from build123d import *

# Parameters (mm, degrees)
F1_DEPTH = 5
F3_DEPTH = 5
F4_R     = 1


with BuildPart() as f1:
    # F0 (on Top) → F1 (new body)
    with BuildSketch(Plane.XY):
        with BuildLine():
            Line((0, 34.5), (0, 32.5))
            ThreePointArc((0, 32.5), (32.5, 0), (0, -32.5))
            Line((0, -32.5), (0, -34.5))
            ThreePointArc((0, -34.5), (34.5, 0), (0, 34.5))
        make_face()
    extrude(amount=F1_DEPTH)

    # F2 (on Top) → F3 (join)
    with BuildSketch(Plane.XY):
        with BuildLine():
            Line((37.856134, -4.425073), (36.986309, -6.22602))
            ThreePointArc((36.986309, -6.22602), (43.716406, 5.833865), (35.63118, -5.362748))
            Line((35.63118, -5.362748), (36.70016, -3.645338))
            ThreePointArc((36.70016, -3.645338), (42.749633, 4.07639), (37.856134, -4.425073))
        make_face()
    extrude(amount=F3_DEPTH)

    # F4
    f4_edges = [f1.edges().sort_by_distance(p)[0] for p in [
        (42.749633, 4.07639, 0),
        (42.749633, 4.07639, 5),
    ]]
    fillet(f4_edges, radius=F4_R)


solid = f1.part
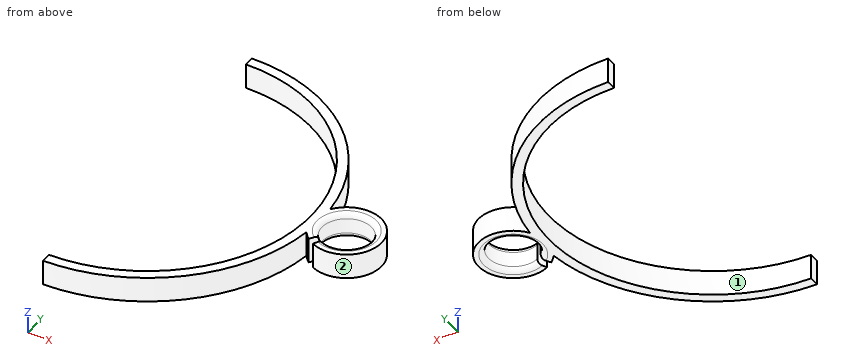
The listing builds one solid part. Answer for the finished solid, in the listing's coordinates (mm). Face numbers are marked on the shaded views. Round coordinates to 2 decimals unless told otherwise and drop trailing zeros. Write each loop counter-clockwise with the first axis right and the second up, starting at its lowest first coordinate (ties: lowest second). Pieces come first, ordered by that corner, then holes. Notation, with made-up numbers: M -30,75 L -20,75 A26 ccw -20,98 Z; hole C 30,2.25 d5. An arc over 180 degrees is marked long. Write each question's results on one line, items separated by ' | '. Start each with the question number.
Item 1: Straight lines are drawn through the part: probe 1 along Y at (x, z) = (40, 2.95); probe 2 along X at (y, z) = (0, 2.65); probe 3 along Y at (x, z) = (4.5, 0.55). For each, find the intervals that lie inside material, in ascending order.
Item 2: The mould has two halves that part along X. Classify the marked faces 1 and 2: +X half, -X half, draft (parallel to the pull), parting line (faces both ways), or undercut.
Item 3: Given pin 1 Ø3 at (y, z) = (-13, 1) entering from -X; pin 2 Ø1.5 at (y, z) = (2.5, 2.5) entering from +X; pin 3 Ø1.5 at (y, z) = (11.5, 2.5) entering from +X, each flat-ended and moving along its own axis, determine where each tip first touches the part or whether it passes through.
Item 4: Find section D-D on y = -15. Write down the section's boundary in (x, z).
Item 5: Find section B-B on z = 3.05. Write down the section's boundary in (x, y).
Item 6: Find section A-A on x = 30. Write down the section's boundary in (y, z).
Item 7: Find section C-C on x = 16. Write down the section's boundary in (y, z), and give its area (3 significant figures).
Answer block:
1) probe 1: y = -6.92 to -4.92, 4.92 to 6.92 | probe 2: x = 32.5 to 35.08, 44.92 to 46.92 | probe 3: y = -34.21 to -32.19, 32.19 to 34.21
2) face 1: -X half | face 2: undercut
3) pin 1: stops at x = 29.09 | pin 2: stops at x = 46.69 | pin 3: stops at x = 32.78
4) outline: M 28.83,0 L 31.07,0 L 31.07,5 L 28.83,5 Z
5) outline: M 0,-34.5 A34.5 ccw 34.28,-3.89 A6.92 ccw 35.63,-5.36 L 36.7,-3.65 A4.92 cw long 37.86,-4.43 L 36.99,-6.23 A6.92 ccw long 34.28,3.89 A34.5 ccw 0,34.5 L 0,32.5 A32.5 cw 0,-32.5 Z
6) outline: M -17.04,0 L -12.5,0 L -12.5,5 L -17.04,5 Z; M 12.5,0 L 17.04,0 L 17.04,5 L 12.5,5 Z
7) outline: M -30.57,0 L -28.29,0 L -28.29,5 L -30.57,5 Z; M 28.29,0 L 30.57,0 L 30.57,5 L 28.29,5 Z | area: 22.8 mm²
